Part model, mm, in its own coordinate system. Give positions to 0.01 mm unless a question says otherwise; leave off trailing zeros. Write each loop counter-clockwise with the first axis right and the second up, starting at its lowest first coordinate (ties: lowest second). Pieces come first, ordered by that corner, then holes. Notation, with made-up numbers: M 2.5,-39.75 L 38.5,-39.75 A28 ccw 38.5,-15.75 Z; hole C 47.5,35.5 d3. An arc over 180 degrees is marked long. Use CSV: the item, a comma, the result in double quotes. Start each with the question number.
1. Band-saw the part on B-B, the plane z = -62.8. List the corners of the cut face in (x, y).
2. Band-saw the part on A-A, the plane x = 0. List the corners of the cut face in (y, z), then the cut area to 3 significant figures.
3. Drill centre lines: line 1 along Z through (x, y) = (-100, 1); line 2 along X through (y, z) = (1.1, -30); line 3 along Z through (x, y) = (0, 1.35). Where is each one in solid material? Low to high. Write a range as from..to.
4. Drop a flat-ended pin along its axis: pin 1 Ø6.5 at (x, z) = (-140, 80) entering from -Y. Give the stop position or say it passes through.
5. Band-saw the part on C-C, the plane y = 1.45. Count the separate pieces of the cut face and the enclosed holes in it, then the cut area to 3 significant figures.
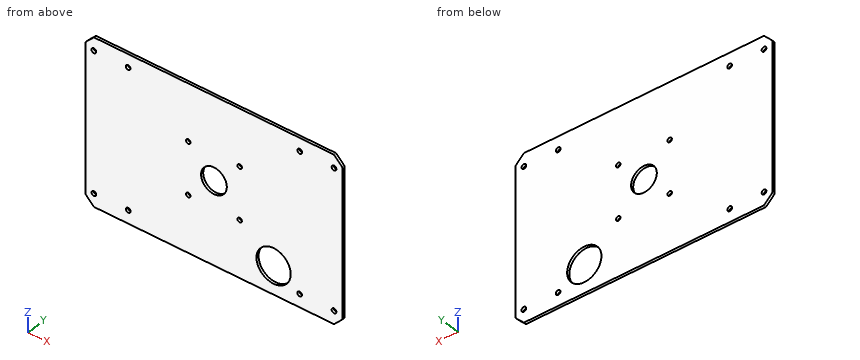
from build123d import *

# Parameters (mm, degrees)
ESQUISSE1_W                     = 300
ESQUISSE1_H                     = 190
BOSS_EXTRU_1_DEPTH              = 3
CHANFREIN1_SIZE                 = 10
CONG_1_R                        = 2
ESQUISSE2_R                     = 2.75
ENL_V_MAT_EXTRU_1_DEPTH         = 4
R_P_TITION_LIN_AIRE1_COUNT      = 2
R_P_TITION_LIN_AIRE1_PITCH      = 240
R_P_TITION_LIN_AIRE1_COUNT_DIR2 = 2
R_P_TITION_LIN_AIRE1_PITCH_DIR2 = 160
ESQUISSE4_R                     = 2.75
ESQUISSE4_R_2                   = 20
ESQUISSE4_R_3                   = 15
ENL_V_MAT_EXTRU_3_DEPTH         = 10
ESQUISSE5_R                     = 2.6
ENL_V_MAT_EXTRU_4_DEPTH         = 4


with BuildPart() as part:
    # Esquisse1 → Boss.-Extru.1 (new body)
    with BuildSketch(Plane(origin=(0, 0, 0), x_dir=(1, 0, 0), z_dir=(0, 1, 0))):
        Rectangle(ESQUISSE1_W, ESQUISSE1_H)
    extrude(amount=BOSS_EXTRU_1_DEPTH)

    # Chanfrein1
    chanfrein1_edges = [part.edges().sort_by_distance(p)[0] for p in [
        (150, 1.5, 95),
        (-150, 1.5, 95),
        (-150, 1.5, -95),
        (150, 1.5, -95),
    ]]
    chamfer(chanfrein1_edges, length=CHANFREIN1_SIZE)

    # Congé1
    cong_1_edges = [part.edges().sort_by_distance(p)[0] for p in [
        (140, 1.5, 95),
        (-140, 1.5, 95),
        (-150, 1.5, -85),
        (-150, 1.5, 85),
        (150, 1.5, -85),
        (150, 1.5, 85),
        (-140, 1.5, -95),
        (140, 1.5, -95),
    ]]
    fillet(cong_1_edges, radius=CONG_1_R)

    # Esquisse2 → Enlèv. mat.-Extru.1 (cut, through all)
    with BuildSketch(Plane.XZ):
        with Locations((-140, 80)):
            Circle(ESQUISSE2_R)
        with Locations((-100, 80)):
            Circle(ESQUISSE2_R)
    enl_v_mat_extru_1 = extrude(amount=-ENL_V_MAT_EXTRU_1_DEPTH, mode=Mode.SUBTRACT)

    # Répétition linéaire1: Enl_v. mat.-Extru.1 2 × 2
    with Locations(*[(i * R_P_TITION_LIN_AIRE1_PITCH, 0, -j * R_P_TITION_LIN_AIRE1_PITCH_DIR2) for i in range(R_P_TITION_LIN_AIRE1_COUNT) for j in range(R_P_TITION_LIN_AIRE1_COUNT_DIR2) if (i, j) != (0, 0)]):
        add(enl_v_mat_extru_1, mode=Mode.SUBTRACT)

    # Esquisse4 → Enlèv. mat.-Extru.3 (cut)
    with BuildSketch(Plane(origin=(0, 3, 0), x_dir=(1, 0, 0), z_dir=(0, 1, 0))):
        with Locations((100, 80)):
            Circle(ESQUISSE4_R)
        with Locations((69.55, 62.8)):
            Circle(ESQUISSE4_R_2)
        Circle(ESQUISSE4_R_3)
    extrude(amount=-ENL_V_MAT_EXTRU_3_DEPTH, mode=Mode.SUBTRACT)

    # Esquisse5 → Enlèv. mat.-Extru.4 (cut, through all)
    with BuildSketch(Plane(origin=(0, 3, 0), x_dir=(1, 0, 0), z_dir=(0, 1, 0))):
        with Locations((-30, 30)):
            Circle(ESQUISSE5_R)
        with Locations((30, 30)):
            Circle(ESQUISSE5_R)
        with Locations((30, -30)):
            Circle(ESQUISSE5_R)
        with Locations((-30, -30)):
            Circle(ESQUISSE5_R)
    extrude(amount=-ENL_V_MAT_EXTRU_4_DEPTH, mode=Mode.SUBTRACT)


solid = part.part
Output:
1,outline,"M -150,0 L 49.55,0 L 49.55,3 L -150,3 Z; M 89.55,0 L 150,0 L 150,3 L 89.55,3 Z"
2,outline,"M 0,-95 L 3,-95 L 3,-15 L 0,-15 Z; M 0,15 L 3,15 L 3,95 L 0,95 Z"
2,area,"480 mm²"
3,line 1,"z = -95..-82.75, -77.25..77.25, 82.75..95"
3,line 2,"x = -150..-32.6, -27.4..27.4, 32.6..150"
3,line 3,"z = -95..-15, 15..95"
4,pin 1,"stops at y = 0"
5,separate pieces,"1"
5,enclosed holes,"14"
5,area,"54,600 mm²"
